Part print with two shaded views. Sizes in mm from the minimum x, y, z corner. A direction names the side the tool comes from. Give positions to 0.01 mm unless a question says otherwise; leave off trailing zeros. Order: outer loops, then holes, each group sorted by start corner. A loop starts at its lowest first (then second) coordinate and runs counter-clockwise, first axis right, second up. Notation, with made-up numbers: M 17,24.25 L 26,24.25 A16 ccw 26,32.25 Z; hole C 18,85.25 d4. An arc over 180 degrees is marked long. Return JSON: item names as keys, results as strings. Group by question number.
1. Pin check, flat tip, straight feed: pin 1 (2 mm diameter, centred on x = 2.5, z = 2.5, fed in from -Y). Stop position of the tip, or through.
2. Slice it at A-A on y = 0.75. List the corners of the cut face in (x, z), then the cut area to 3 significant figures.
3. Wall check: probe 1 along Z at (x, y) = (7.5, 0.65); probe 2 along Z at (x, y) = (7, 2.3); probe 3 along Z at (x, y) = (8.25, 0.45). Give the ranges that are in metal, low to high. Write a range as [from, to].
4. 3-axis set-ups, long thin cutter, end or side, ignore diameter. For the marked faces 1, 2 and 3: which of +Z, -Z, +X, -X, +Y, -Y reach the whole face in a straight line?
5. Slice it at B-B on x = 2.5. List the corners of the cut face in (y, z).
6. Slice it at C-C on z = 12.5. List the corners of the cut face in (x, y), then the cut area to 3 significant figures.
7. Slice it at D-D on y = 2.65. List the corners of the cut face in (x, z).
8. Two-plate mould, pull along Z, no slides. Class the marked faces 4, 5 and 6: released by +Z, released by -Z, zero draft, split by the parting line, or undercut.
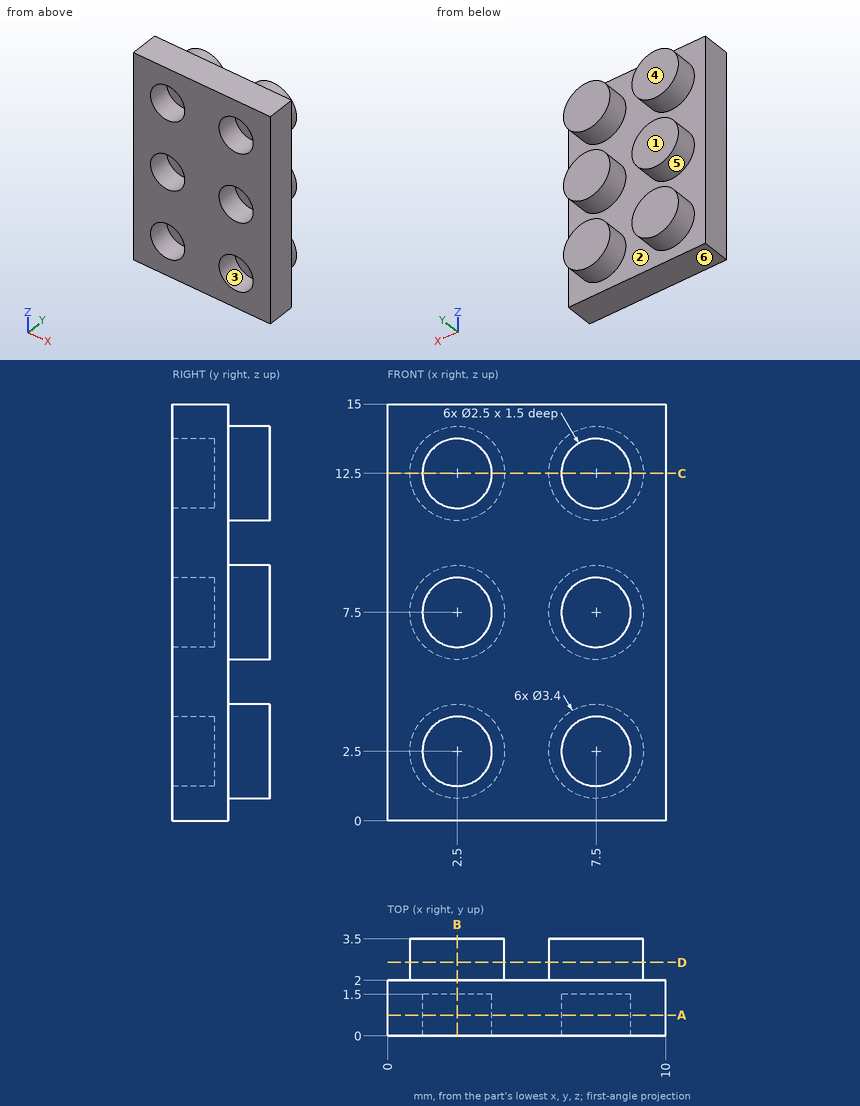
Result:
{
 "1": {"pin 1": "stops at y = 1.5"},
 "2": {"outline": "M 0,0 L 10,0 L 10,15 L 0,15 Z; hole C 2.5,2.5 d2.5; hole C 2.5,7.5 d2.5; hole C 2.5,12.5 d2.5; hole C 7.5,2.5 d2.5; hole C 7.5,7.5 d2.5; hole C 7.5,12.5 d2.5", "area": "121 mm2"},
 "3": {"probe 1": "z = [0, 1.25], [3.75, 6.25], [8.75, 11.25], [13.75, 15]", "probe 2": "z = [0.88, 4.12], [5.88, 9.12], [10.88, 14.12]", "probe 3": "z = [0, 1.5], [3.5, 6.5], [8.5, 11.5], [13.5, 15]"},
 "4": {"face 1": "+Z, -Z, +X, -X, +Y", "face 2": "+Y", "face 3": "-Y"},
 "5": {"outline": "M 0,0 L 2,0 L 2,0.8 L 3.5,0.8 L 3.5,4.2 L 2,4.2 L 2,5.8 L 3.5,5.8 L 3.5,9.2 L 2,9.2 L 2,10.8 L 3.5,10.8 L 3.5,14.2 L 2,14.2 L 2,15 L 0,15 L 0,13.75 L 1.5,13.75 L 1.5,11.25 L 0,11.25 L 0,8.75 L 1.5,8.75 L 1.5,6.25 L 0,6.25 L 0,3.75 L 1.5,3.75 L 1.5,1.25 L 0,1.25 Z"},
 "6": {"outline": "M 0,0 L 1.25,0 L 1.25,1.5 L 3.75,1.5 L 3.75,0 L 6.25,0 L 6.25,1.5 L 8.75,1.5 L 8.75,0 L 10,0 L 10,2 L 9.2,2 L 9.2,3.5 L 5.8,3.5 L 5.8,2 L 4.2,2 L 4.2,3.5 L 0.8,3.5 L 0.8,2 L 0,2 Z", "area": "22.7 mm2"},
 "7": {"outline": "C 2.5,2.5 d3.4; C 2.5,7.5 d3.4; C 2.5,12.5 d3.4; C 7.5,2.5 d3.4; C 7.5,7.5 d3.4; C 7.5,12.5 d3.4"},
 "8": {"face 4": "zero draft", "face 5": "undercut", "face 6": "released by -Z"}
}
